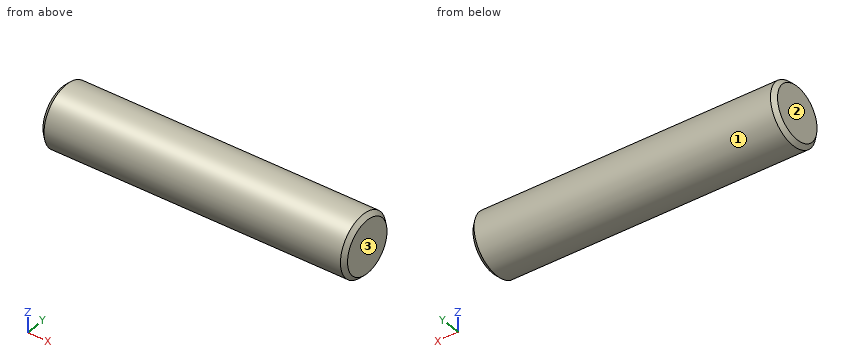
Autodesk Inventor part; units mm, degrees
ref_plane "Work Plane1" through (15, 0, 0) normal (1, 0, 0) x (0, 1, 0)
ref_plane "YZ Plane" through (0, 0, 0) normal (1, 0, 0) x (0, 1, 0)
ref_plane "XZ Plane" through (0, 0, 0) normal (0, 1, 0) x (-1, 0, 0)
sketch "Sketch1" plane through (0, 0, 0) normal (0, 0, 1) x (1, 0, 0)
  line L0 (0, 0) -> (0, 6)
  line L1 (0, 6) -> (15, 6)
  line L2 (15, 6) -> (15, 6)
  line L3 (15, 6) -> (30, 6)
  line L4 (30, 6) -> (30, 6)
  line L5 (30, 6) -> (60, 6)
  line L6 (60, 6) -> (60, 0)
  line L7 (60, 0) -> (0, 0)
  dimension "d1" = 12
  dimension "d3" = 12
  dimension "d4" = 15
  dimension "d5" = 45
  dimension "d6" = 30
revolve "Revolution1" add sketch "Sketch1" angle 360 about axis through (60, 0, 0) along (-1, 0, 0)
thread "Thread1"
thread "Thread2"
chamfer "Chamfer1" distance 0.8 angle 45 2 edges at (60, -6, 0) (0, -6, 0)
ref_plane "Work Plane1" through (15, 0, 0) normal (1, 0, 0) x (0, 1, 0)
sketch "Sketch2" plane through (15, 0, 0) normal (1, 0, 0) x (0, 1, 0)
  circle A0 centre (0, 0) radius 6
  point P0 (0, 0)
  dimension "d29" = 12
boundary_patch "Boundary Patch1"
equation "\"d8\" = d4"
equation "\"d23\" = b"
equation "\"d25\" = chamfer"
equation "\"d1\" = d"
equation "\"d3\" = d1_"
equation "\"d4\" = b1"
equation "\"d5\" = L"
equation "\"d6\" = b"
equation "\"d29\" = d"
equation "\"chamfer\" = 0.8"
equation "\"d\" = 12"
equation "\"d1_\" = 12"
equation "\"b1\" = 15"
equation "\"L\" = 45"
equation "\"b\" = 30"
equation "\"d28\" = -b1"
equation "\"Grip_Length\" = 15"
properties part number "Stud M12-6g×45 GOST 22034-76" material "Steel, Mild"
CAD build for the part. Positions are in the model's coordinates, mm. Face numbers are marked on the shaded views. Give positions to 0.01 mm unless a question says otherwise; leave off trailing zeros. Write each loop counter-clockwise with the first axis right and the second up, starting at its lowest first coordinate (ties: lowest second). Pieces come first, ordered by that corner, then holes. Notation, with made-up numbers: (7, -36.75) -> (61, -36.75) arc R16 ccw to (61, -16.75) -> close; hole circle Ø1 at (16, 4). An arc over 180 degrees is marked (long way). Write each question's results on one line, items separated by ' | '.
1. Two-plate mould, pull along X, no slides. Class the marked faces 1, 2 and 3: pulls with the +X half, pulls with the -X half, needs draft (parallel to the pull), parting line crosses it, or undercut.
Geometry check:
face 1: needs draft | face 2: pulls with the -X half | face 3: pulls with the +X half
2. Wall check: probe 1 along Y at (x, z) = (18, -0.25); probe 2 along Y at (x, z) = (37.5, 3); probe 3 along Z at (x, y) = (26, 1.5). Give the ranges that are in metal, low to high. Write a range as [from, to].
Geometry check:
probe 1: [-5.99, 5.99] | probe 2: [-5.2, 5.2] | probe 3: [-5.81, 5.81]
3. Drop flat-ended pins along their axis: P1, Ø1.5, axis at x = 45.5, z = -2.5, coming from the -Y side; P2, Ø3, axis at x = 45.5, z = 3, coming from the +Y side. Give the stop position or say it passes through.
Geometry check:
P1: y = -5.74 | P2: y = 5.81
4. Cut at A-A, the plane x = 14. Write the cut outline in (y, z).
Geometry check:
outline: circle Ø12 at (0, 0)
